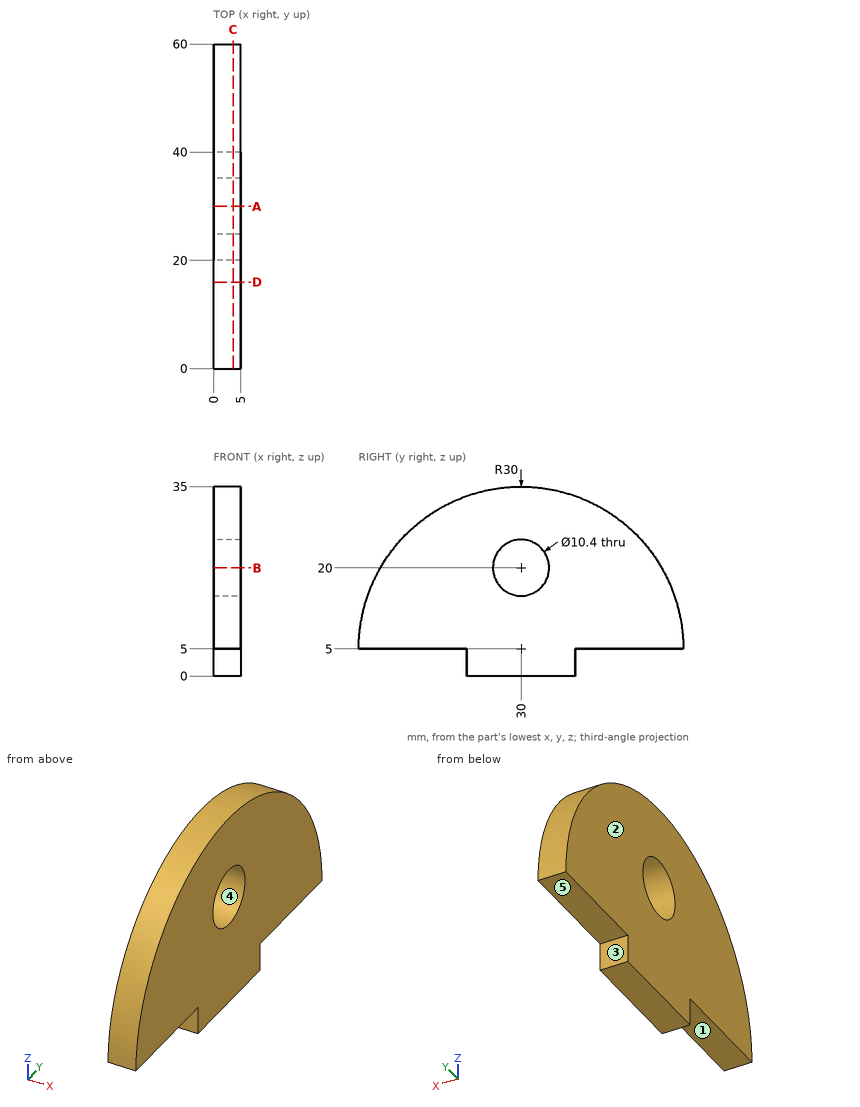
Check sheet for the drawn part. Datum: minimum x, y, z corner. Units: mm. A direction names the side the tool comes from. Coordinates: 2 decimals unless noted, no trailing zeros. Loops run counter-clockwise (first coordinate to the right, second up) from the corner with the lowest first, then second, coordinate; pieces in that order, holes last. Notation, with made-up numbers: (-39.75, -14.75) -> (-23.75, -14.75) arc R13 cw to (-23.75, 5.25) -> close; hole circle Ø7 at (64.5, 29.25). An arc over 180 degrees is marked (long way). Answer in a Markdown table with one row per item.
1) Section check C-C (x = 3.6). Record the cut outline in (y, z), and give its area (3 significant figures).
The answers:
| item | result |
|---|---|
| outline | (0, 5) -> (20, 5) -> (20, 0) -> (40, 0) -> (40, 5) -> (60, 5) arc R30 ccw to start; hole circle Ø10.4 at (30, 20) |
| area | 1,430 mm2 |
2) Depth check by flat-ended pin: P1, Ø3, axis at x = 2, y = 51, coming from the +Z side; P2, Ø1.5, axis at x = 2.5, z = 3, coming from the -Y side; P3, Ø2.5, axis at x = 1.5, y = 11, coming from the -Z side. Enter the tip coordinate at first touch or a pass-through.
The answers:
| item | result |
|---|---|
| P1 | stops at z = 27.8 |
| P2 | stops at y = 20 |
| P3 | stops at z = 5 |
3) Access from +Z, -Z, +X, -X, +Y, -Y to the whole of each face (thin tool, end or side, straight path). Record for the marked faces 1 and 2.
The answers:
| item | result |
|---|---|
| face 1 | -Z, +X, -X, -Y |
| face 2 | +Z, -Z, -X, +Y, -Y |
4) Section check D-D (y = 16). Record the cut outline in (x, z), and give its area (3 significant figures).
The answers:
| item | result |
|---|---|
| outline | (0, 5) -> (5, 5) -> (5, 31.53) -> (0, 31.53) -> close |
| area | 133 mm2 |
5) Section check B-B (z = 20). Record the cut outline in (x, y).
The answers:
| item | result |
|---|---|
| outline | (0, 4.02) -> (5, 4.02) -> (5, 24.8) -> (0, 24.8) -> close; (0, 35.2) -> (5, 35.2) -> (5, 55.98) -> (0, 55.98) -> close |
6) Scan lines: line 1 along Y through (x, z) = (2.15, 20); line 2 along Y through (x, z) = (3.05, 20.5); line 3 along Z through (x, y) = (1.55, 27). Record each from-to range of solid material in increasing order. Write a range as from..to.
The answers:
| item | result |
|---|---|
| line 1 | y = 4.02..24.8, 35.2..55.98 |
| line 2 | y = 4.31..24.82, 35.18..55.69 |
| line 3 | z = 0..15.75, 24.25..34.85 |
7) Section check A-A (y = 30). Record the cut outline in (x, z), and give its area (3 significant figures).
The answers:
| item | result |
|---|---|
| outline | (0, 0) -> (5, 0) -> (5, 14.8) -> (0, 14.8) -> close; (0, 25.2) -> (5, 25.2) -> (5, 35) -> (0, 35) -> close |
| area | 123 mm2 |
8) Draft check along Z on the marked faces 3, 4 and 5. Enter one of: released by +Z, released by -Z, zero draft, split by the parting line, or undercut.
The answers:
| item | result |
|---|---|
| face 3 | zero draft |
| face 4 | undercut |
| face 5 | released by -Z |
